Autodesk Inventor part; units mm, degrees
ref_plane "Work Plane1" through (19.05, 73.7803, 37.8333) normal (0, 1, 0) x (-1, 0, 0)
ref_plane "Work Plane2" through (0, 197.6053, 37.8333) normal (0, 1, 0) x (-1, 0, 0)
ref_plane "YZ Plane" through (0, 0, 0) normal (1, 0, 0) x (0, 1, 0)
sketch "Sketch1" plane through (0, 0, 0) normal (0, 0, 1) x (1, 0, 0)
  arc A0 (19.05, 73.7803) -> (-19.05, 73.7803) centre (0, 0) ccw
  line L0 (0, 86.4803) -> (19.05, 86.4803)
  line L1 (19.05, 86.4803) -> (19.05, 73.7803)
  line L2 (0, 76.2) -> (0, 86.4803) construction
  line L3 (0, 86.4803) -> (-19.05, 86.4803)
  line L4 (-19.05, 86.4803) -> (-19.05, 73.7803)
  dimension "d0" = 152.4
  dimension "d1" = 19.05
  dimension "d2" = 12.7
extrude "Extrusion1" add sketch "Sketch1" along normal mid plane 75.6666
sketch "Sketch2" plane through (-19.05, 86.4803, 37.8333) normal (0, 1, 0) x (1, 0, 0)
  line L0 (0, 75.6666) -> (0, 0) construction
  line L1 (0, 37.8333) -> (38.1, 37.8333) construction
  line L2 (38.1, 75.6666) -> (38.1, 0) construction
  line L3 (0, 75.6666) -> (38.1, 75.6666) construction
  line L4 (19.05, 75.6666) -> (19.05, 0) construction
  line L5 (38.1, 0) -> (0, 0) construction
  line L6 (28.575, 34.3408) -> (28.575, 41.3258) construction
  line L7 (24.4475, 34.3408) -> (24.4475, 41.3258)
  line L8 (32.7025, 41.3258) -> (32.7025, 34.3408)
  arc A0 (24.4475, 34.3408) -> (32.7025, 34.3408) centre (28.575, 34.3408) ccw
  arc A1 (32.7025, 41.3258) -> (24.4475, 41.3258) centre (28.575, 41.3258) ccw
  line L9 (13.6525, 34.3408) -> (13.6525, 41.3258)
  line L10 (5.3975, 41.3258) -> (5.3975, 34.3408)
  arc A2 (5.3975, 34.3408) -> (13.6525, 34.3408) centre (9.525, 34.3408) ccw
  arc A3 (13.6525, 41.3258) -> (5.3975, 41.3258) centre (9.525, 41.3258) ccw
  point P0 (19.05, 37.8333)
  point P1 (28.575, 37.8333)
  dimension "d5" = 9.525
  dimension "d6" = 8.255
  dimension "d7" = 15.24
  dimension "d8" = 19.05
  dimension "d170" = 8.255
extrude "Extrusion2" cut sketch "Sketch2" against normal through all
ref_plane "Work Plane1" through (19.05, 73.7803, 37.8333) normal (0, 1, 0) x (-1, 0, 0)
sketch "Sketch5" plane through (0, 0, 37.8333) normal (0, 0, 1) x (1, 0, 0)
  circle A0 centre (0, 175.3803) radius 15.875
  arc A1 (9.525, 155.2999) -> (-9.525, 155.2999) centre (0, 175.3803) ccw
  arc A2 (19.05, 73.7803) -> (-19.05, 73.7803) centre (0, 0) ccw construction
  line L0 (-19.05, 73.7803) -> (19.05, 73.7803) construction
  line L1 (19.05, 86.4803) -> (9.525, 155.2999)
  line L2 (19.05, 86.4803) -> (-19.05, 86.4803) construction
  line L3 (0, 86.4803) -> (0, 175.3803) construction
  line L4 (-19.05, 86.4803) -> (-9.525, 155.2999)
  line L5 (-19.05, 86.4803) -> (19.05, 86.4803)
  dimension "d15" = 31.75
  dimension "d16" = 6.35
  dimension "d17" = 101.6
  dimension "d18" = 9.525
extrude "Extrusion4" add sketch "Sketch5" against normal blind 9.525
ref_plane "Work Plane2" through (0, 197.6053, 37.8333) normal (0, 1, 0) x (-1, 0, 0)
sketch "Sketch6" plane through (0, 197.6053, 37.8333) normal (0, 1, 0) x (-1, 0, 0)
  line L0 (-22.225, -9.525) -> (22.225, -9.525)
  circle A0 centre (0, -4.7625) radius 1.7272
  point P0 (0, -37.8333)
  point P1 (9.525, -9.525)
  point P2 (-9.525, -9.525)
  dimension "d21" = 4.7625
  dimension "d22" = 3.4544
extrude "Extrusion5" cut sketch "Sketch6" against normal up to surface
pattern_circular "Circular Pattern1" count 3 over 360 about axis through (0, 175.3803, 37.8333) along (0, 0, -1) of "Extrusion5"
mirror "Mirror1" about plane through (0, 0, 0) normal (0, 0, 1) of "Extrusion4", "Extrusion5", "Circular Pattern1"
sketch "Sketch20" plane through (19.05, 73.7803, 37.8333) normal (1, 0, 0) x (0, 0, -1)
  line L0 (0, 12.7) -> (0, 0)
  line L1 (75.6666, 12.7) -> (75.6666, 0)
  line L2 (0, 0) -> (75.6666, 0)
  line L3 (75.6666, 0) -> (75.6666, 6.35)
  line L4 (75.6666, 6.35) -> (0, 6.35)
  line L5 (0, 6.35) -> (0, 0)
  point P0 (37.8333, -73.7803)
  point P1 (0, 6.35)
extrude "Extrusion7" cut sketch "Sketch20" against normal through all
sketch "Sketch22" plane through (-19.05, 86.4803, 28.3083) normal (0, 1, 0) x (1, 0, 0)
  line L0 (41.275, 0) -> (-3.175, 0)
  line L1 (41.275, 56.6166) -> (-3.175, 56.6166)
  line L2 (-3.175, 66.1416) -> (41.275, 66.1416)
  point P0 (19.05, 28.3083)
  point P1 (19.05, 6.35)
  point P2 (19.05, 50.2666)
  point P3 (9.525, 0)
  point P4 (28.575, 0)
  point P5 (9.525, 56.6166)
  point P6 (28.575, 56.6166)
  point P7 (28.575, 66.1416)
  point P8 (9.525, 66.1416)
  dimension "d173" = 6.35
  dimension "d174" = 6.35
  dimension "d183" = 15.875
hole "Hole1" at (0, 86.4803, 21.9583) at (0, 86.4803, -21.9583) direction (0, -1, 0) diameter 5.1054 end through all
equation "\"d51\" = 0.125 * Sketch8_Pitch"
equation "\"Sketch8_Pitch\" = 0.79375"
equation "\"d53\" = 60deg"
equation "\"d72\" = 0.125 * Sketch10_Pitch"
equation "\"Sketch10_Pitch\" = 0.79375"
equation "\"d74\" = 60deg"
equation "\"d93\" = 0.125 * Sketch12_Pitch"
equation "\"Sketch12_Pitch\" = 0.79375"
equation "\"d95\" = 60deg"
equation "\"d114\" = 0.125 * Sketch14_Pitch"
equation "\"Sketch14_Pitch\" = 0.79375"
equation "\"d116\" = 60deg"
equation "\"d135\" = 0.125 * Sketch16_Pitch"
equation "\"Sketch16_Pitch\" = 0.79375"
equation "\"d137\" = 60deg"
equation "\"d156\" = 0.125 * Sketch18_Pitch"
equation "\"Sketch18_Pitch\" = 0.79375"
equation "\"d158\" = 60deg"
properties part number "finderMainPartV05"
The model under review builds one solid part; all positions refer to its coordinate system, in mm. A direction names the side the tool comes from. Coordinates: 2 decimals unless noted, no trailing zeros. Write each loop counter-clockwise with the first axis right and the second up, starting at its lowest first coordinate (ties: lowest second). Pieces come first, ordered by that corner, then holes. Notation, with made-up numbers: (-6, -2.5) - (-2, -2.5) arc R23 ccw to (-2, 28.5) - close; hole circle Ø3 at (-31.5, -19.5). An arc over 180 degrees is marked (long way). Write item = value, one per line.
(1) Mouldability with a two-part tool opening along Y and no side actions: class faces 4 (the face through (9.62, 83.35, -7.62)), 5 (the face through (-15.67, 164.43, -32.55)) as pulls with the +Y half, pulls with the -Y half, needs draft (parallel to the pull), parting line crosses it, or undercut.
Result sheet:
face_4 = needs draft
face_5 = undercut
(2) Consider section B-B, the plane z = 0. Give the boundary of the cut face in (x, y), then the cut area to 3 significant figures.
Result sheet:
outline = (-19.05, 80.13) - (-13.65, 80.13) - (-13.65, 86.48) - (-19.05, 86.48) - close; (-5.4, 80.13) - (5.4, 80.13) - (5.4, 86.48) - (-5.4, 86.48) - close; (13.65, 80.13) - (19.05, 80.13) - (19.05, 86.48) - (13.65, 86.48) - close
area = 137 mm^2
(3) Consider section C-C, the plane y = 115.5. Give the boundary of the cut face in (x, z), then the cut area to 3 significant figures.
Result sheet:
outline = (-15.03, -37.83) - (15.03, -37.83) - (15.03, -28.31) - (-15.03, -28.31) - close; (-15.03, 28.31) - (15.03, 28.31) - (15.03, 37.83) - (-15.03, 37.83) - close
area = 573 mm^2
(4) For P1, Ø11.5, axis at x = -1, z = -13, coming from the +Y side; P2, Ø5, axis at y = 81.5, z = -1.5, coming from the +X side; P3, Ø3, axis at y = 82, z = 0.5, coming from the -X side, all flat-tipped, find the tip position at first contact; note any pin that passes through.
Result sheet:
P1 = 86.48
P2 = 19.05
P3 = -19.05
(5) Consider section D-D, the plane z = -22.5. Give the boundary of the cut face in (x, y), then the cut area to 3 significant figures.
Result sheet:
outline = (-19.05, 80.13) - (-2.49, 80.13) - (-2.49, 86.48) - (-19.05, 86.48) - close; (2.49, 80.13) - (19.05, 80.13) - (19.05, 86.48) - (2.49, 86.48) - close
area = 210 mm^2
(6) For line 1 (Z direction, x = 0, y = 196); line 2 (Z direction, x = 0, y = 85); line 3 (Z direction, x = -2.5, y = 101), list the stretches that pass through material, from the lowest coordinate up. Write a range as [from, to].
Result sheet:
line_1 = [-37.83, -34.8], [-31.34, -28.31], [28.31, 31.34], [34.8, 37.83]
line_2 = [-37.83, -24.51], [-19.41, 19.41], [24.51, 37.83]
line_3 = [-37.83, -28.31], [28.31, 37.83]
(7) Machinability: for faces 1 (the face through (0, 130, 28.308)), 2 (the face through (14.22, 121.37, -33.14)), 3 (the face through (5.398, 83, 0)), which of the approach directions +Z, -Z, +X, -X, +Y, -Y give a long, thin tool a straight path to every point of the face, cutting with its end or side? Answer none if there is none.
Result sheet:
face_1 = +X, -X, +Y
face_2 = +Z, -Z, +X
face_3 = +Y, -Y
(8) Consider section A-A, the plane x = 0. State how many separate pieces and enclosed holes the cut face has, then the cut area to 3 significant figures.
Result sheet:
separate_pieces = 7
enclosed_holes = 0
area = 1,880 mm^2
